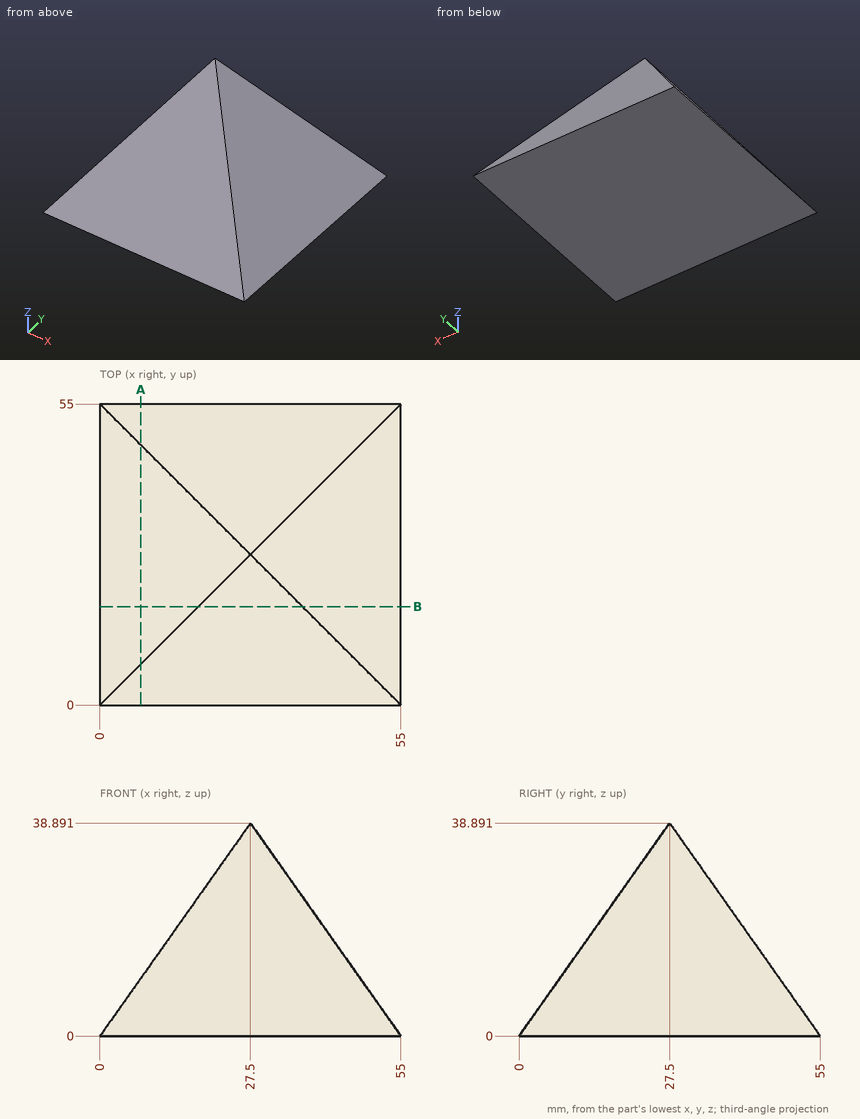
Could you check a few things on this drawing? It's one solid part, dimensions in mm from its lowest x, y, z. Coordinates: 2 decimals unless noted, no trailing zeros. Order: outer loops, then holes, each group sorted by start corner. A loop starts at its lowest first (then second) coordinate and runs counter-clockwise, first axis right, second up.
1. If we section it at A-A (x = 7.5): Please give me the cut outline in (y, z).
2. I need wall thicknesses on line 1 (Z direction, x = 20.5, y = 20.5); line 2 (Y direction, x = 33.5, z = 5.5); line 3 (X direction, y = 11, z = 11.5). Which ranges of each line are inside material? Lowest first, please.
3. I'm going to push flat-ended pins straight in: pin 1 (5 mm diameter, centred on x = 23.5, z = 26, fed in from -Y); pin 2 (10 mm diameter, centred on x = 49, z = 11, fed in from +Y); pin 3 (10 mm diameter, centred on x = 13, y = 24.5, fed in from +Z); pin 4 (3 mm diameter, centred on x = 6, z = 14.5, fed in from -Y). Where does each tip first touch, or does it pass through?
4. If we section it at B-B (y = 18): Please give me the cut outline in (x, z).
Entries:
1. outline: (0, 0) - (55, 0) - (47.5, 10.61) - (7.5, 10.61) - close
2. line 1: z = 0 to 28.99
2. line 2: y = 3.89 to 51.11
2. line 3: x = 8.13 to 46.87
3. pin 1: stops at y = 16.62
3. pin 2: stops at y = 50.76
3. pin 3: stops at z = 25.46
3. pin 4: passes through
4. outline: (0, 0) - (55, 0) - (37, 25.46) - (18, 25.46) - close
